Design review of the part built by this model. Coordinates are the model's own, in mm. A direction names the side the tool comes from. Round coordinates to 2 decimals unless told otherwise and drop trailing zeros. Order: outer loops, then holes, each group sorted by start corner. A loop starts at its lowest first (then second) coordinate and runs counter-clockwise, first axis right, second up. Notation, with made-up numbers: M 64.5,-21.75 L 72.5,-21.75 A21 ccw 72.5,10.25 Z; hole C 50,65.5 d1. An arc over 180 degrees is marked long. Write item = value, one per line. Start each with the question number.
Autodesk Inventor part; units mm, degrees
ref_plane "YZ Plane" through (0, 0, 0) normal (1, 0, 0) x (0, 1, 0)
ref_plane "XZ Plane" through (0, 0, 0) normal (0, 1, 0) x (-1, 0, 0)
ref_plane "XY Plane" through (0, 0, 0) normal (0, 0, 1) x (1, 0, 0)
sketch "Sketch1" plane through (0, 0, 0) normal (0, 0, 1) x (1, 0, 0)
  line L0 (0, 0) -> (-4, 0)
  line L1 (-4, 0) -> (-4, -6.15)
  line L2 (-4, -6.15) -> (0, -6.15)
  line L3 (0, -6.15) -> (0, 0)
  line L4 (0, 0) -> (-13.1356, 0) construction
  dimension "d1" = 6.15
  dimension "d2" = 4
revolve "Shoulder" add sketch "Sketch1" angle 360 about axis through (0, -6.15, 0) along (0, 1, 0)
sketch "Sketch2" plane through (0, 0, 0) normal (0, 1, 0) x (1, 0, 0)
  circle A0 centre (0, 0) radius 4
  circle A1 centre (0, 0) radius 3.76
  dimension "d3" = 7.52
extrude "Shoulder_neck" add sketch "Sketch2" along normal blind 1.85 contours A1
sketch "Sketch3" plane through (0, 1.85, 0) normal (0, 1, 0) x (1, 0, 0)
  circle A0 centre (0, 0) radius 3.76
  circle A1 centre (0, 0) radius 6.6
  dimension "d6" = 13.2
extrude "Head" add sketch "Sketch3" along normal blind 5.5 contours A0 | A1
sketch "Sketch4" plane through (0, -6.15, 0) normal (0, -1, 0) x (1, 0, 0)
  circle A0 centre (0, 0) radius 4
  circle A1 centre (0, 0) radius 2.255
  dimension "d9" = 4.51
extrude "Thread_neck" add sketch "Sketch4" along normal blind 2.3 contours A1
sketch "Sketch5" plane through (0, -8.45, 0) normal (0, -1, 0) x (1, 0, 0)
  circle A0 centre (0, 0) radius 2.255
  circle A1 centre (0, 0) radius 3
  dimension "d12" = 6
extrude "Thread_shoulder" add sketch "Sketch5" along normal blind 8.7 contours A0 | A1
sketch "Sketch6" plane through (0, 7.35, 0) normal (0, 1, 0) x (1, 0, 0)
  circle A0 centre (0, 0) radius 6.6
  circle A1 centre (0, 0) radius 2 construction
  line L0 (-2, 1.1547) -> (-2, -1.1547)
  line L1 (-2, -1.1547) -> (0, -2.3094)
  line L2 (0, -2.3094) -> (2, -1.1547)
  line L3 (2, -1.1547) -> (2, 1.1547)
  line L4 (2, 1.1547) -> (0, 2.3094)
  line L5 (0, 2.3094) -> (-2, 1.1547)
  dimension "d15" = 4
extrude "Hex" cut sketch "Sketch6" against normal blind 3.3 contours L5 L4 L3 L2 L1 L0
chamfer "Chamfer1" distance 0.24 angle 30 1 edges at (4, 0, 0) measured on face at (-3.8813, 0, -0.3191)
fillet "Fillet1" radius 0.4 1 edges at (-3.76, 1.85, 0)
chamfer "Chamfer2" distance 0.4 angle 30 1 edges at (-6.6, 7.35, 0) measured on face at (6.5145, 5.5167, 1.0587)
chamfer "Chamfer3" distance 0.5 angle 30 1 edges at (-3, -17.15, 0) measured on face at (-0.5351, -17.15, 1.0949)
fillet "Fillet2" radius 0.6 1 edges at (-2.255, -6.15, 0)
chamfer "Chamfer7" distance 0.745 angle 30 1 edges at (-3, -8.45, 0) measured on face at (2.7226, -8.45, -0.2393)
thread "Thread"
equation "\"d3\" = Shoulder_neck_dia"
equation "\"d4\" = Shoulder_neck_length"
equation "\"d6\" = Head_diameter"
equation "\"d7\" = Head_height"
equation "\"d9\" = Thread_neck_dia"
equation "\"d10\" = Thread_neck_length"
equation "\"d12\" = Thread_diameter"
equation "\"d13\" = Thread_length - Thread_neck_length"
equation "\"d15\" = Hex_size"
equation "\"d16\" = Hex_length"
equation "\"d18\" = -0.5 * Shoulder_neck_dia + 0.5 * Shoulder_diameter"
equation "\"d64\" = -0.5 * Shoulder_neck_dia + 0.5 * Shoulder_diameter"
equation "\"d21\" = 0.1 * Hex_size"
equation "\"d65\" = 0.1 * Hex_size"
equation "\"d23\" = 0.5 * Thread_pitch"
equation "\"d66\" = 0.5 * Thread_pitch"
equation "\"d25\" = Thread_neck_radius"
equation "\"d60\" = -0.5 * Thread_neck_dia + 0.5 * Thread_diameter"
equation "\"d67\" = -0.5 * Thread_neck_dia + 0.5 * Thread_diameter"
equation "\"d1\" = Shoulder_length - Shoulder_neck_length"
equation "\"d2\" = 0.5 * Shoulder_diameter"
equation "\"Shoulder_diameter\" = 8"
equation "\"Shoulder_length\" = 8"
equation "\"Shoulder_neck_dia\" = 7.52"
equation "\"Thread_diameter\" = 6"
equation "\"Thread_length\" = 11"
equation "\"Head_diameter\" = 13.2"
equation "\"Head_height\" = 5.5"
equation "\"Thread_neck_dia\" = 4.51"
equation "\"Hex_size\" = 4"
equation "\"Hex_length\" = 3.3"
equation "\"Thread_pitch\" = 1"
equation "\"Shoulder_neck_length\" = 1.85"
equation "\"Thread_neck_length\" = 2.3"
equation "\"Thread_neck_radius\" = 0.6"
properties part number "SCREW,SHOULDER,M8X8MM" material "Steel, High Strength Low Alloy"
(1) Consider section A-A, the plane y = 4.5. Write out the cut boundary in (x, z), then the cut area to 3 significant figures.
(2) Insertion check: pin 1 (2 mm diameter, centred on y = -10, z = -2.5, fed in from +X); pin 2 (2 mm diameter, centred on x = 0, z = 0.5, fed in from +Y); pin 3 (6 mm diameter, centred on x = -3.5, y = -14, fed in from +Z). Each pin has a flat end and moves straight along its axis. Give the tip position at first contact, or say it passes through.
(3) For faces 4 (the face through (-2, 7.35, -2)), 5 (the face through (-0.99, 5.72, -1.74)), 6 (the face through (3.586, 0.715, 1.129)), 7 (the face through (-3, -13, 0)), list the 3-axis set-ups (+Z, -Z, +X, -X, +Y, -Y) from which the entire face can be reached by the end or side of a thin tool; tool diameter is ignored.
(4) Consider section C-C, the plane y = -7.5. Write out the cut boundary in (x, z) (3 decimals), then the cut area to 3 significant figures.
(5) Draft analysis for pull direction Y (two halves, no side actions). For faces 1 (the face through (2.083, -7.588, 0.864)), 2 (the face through (0.99, 5.72, 1.74)), 3 (the face through (0, 4.05, 0)), state which applies: pulls with the +Y half, pulls with the -Y half, needs draft (parallel to the pull), parting line crosses it, or undercut.
(6) Consider section B-B, the plane y = -15.25. Write out the cut boundary in (x, z), then the cut area to 3 significant figures.
(7) For line 1 along Y through (x, z) = (4, -2.5); line 2 along Y through (x, z) = (-0.75, -2.25); line 3 along X through (y, z) = (5.25, 0.5), list the stretches that pass through material, from the lowest coordinate up. Write a range as [from, to].
Completed:
q1.outline = C 0,0 d13.2; hole M -2,-1.15 L 0,-2.31 L 2,-1.15 L 2,1.15 L 0,2.31 L -2,1.15 Z
q1.area = 123 mm2
q2.pin_1 = 2.6
q2.pin_2 = 4.05
q2.pin_3 = 2.96
q3.face_4 = +Z, -Z, +X, -X, +Y
q3.face_5 = +Y
q3.face_6 = none
q3.face_7 = -Y
q4.outline = C 0,0 d4.51
q4.area = 16.0 mm2
q5.face_1 = undercut
q5.face_2 = needs draft
q5.face_3 = pulls with the +Y half
q6.outline = C 0,0 d6
q6.area = 28.3 mm2
q7.line_1 = [1.85, 7.35]
q7.line_2 = [-17.15, -8.52], [-6.39, 7.35]
q7.line_3 = [-6.58, -2], [2, 6.58]
